Here's how the part is built. I have some questions about the finished solid (model axes, mm). A direction names the side the tool comes from. Give positions to 0.01 mm unless a question says otherwise; leave off trailing zeros. Loops run counter-clockwise (first coordinate to the right, second up) from the corner with the lowest first, then second, coordinate; pieces in that order, holes last. Notation, with made-up numbers: (41.5, 51.5) - (59.5, 51.5) arc R17 ccw to (59.5, 62.5) - close; hole circle Ø2 at (-24.5, -8.5). An arc over 180 degrees is marked (long way). Put each result on its own line as item: value. Start each with the question number.
from build123d import *

# Parameters (mm, degrees)
SKETCH1_R           = 2.5
BOSS_EXTRUDE1_DEPTH = 1
SKETCH2_R           = 1.57
BOSS_EXTRUDE2_DEPTH = 1
BOSS_EXTRUDE3_START = 11
SKETCH3_R           = 2.5
BOSS_EXTRUDE3_DEPTH = 11
SKETCH4_R           = 3
BOSS_EXTRUDE4_DEPTH = 16
SKETCH6_R           = 3.5
BOSS_EXTRUDE6_DEPTH = 8
SKETCH7_W           = 8.052083516
SKETCH7_H           = 1.294876405
CUT_EXTRUDE1_DEPTH  = 30.419381367
SKETCH8_R           = 3.5
BOSS_EXTRUDE7_DEPTH = 29
CUT_EXTRUDE2_START  = -18
SKETCH9_R           = 3
CUT_EXTRUDE2_DEPTH  = 18
SKETCH10_W          = 13
SKETCH10_H          = 5.291502622
CUT_EXTRUDE3_DEPTH  = 3
SKETCH11_R          = 9
BOSS_EXTRUDE8_DEPTH = 4
CUT_EXTRUDE4_START  = -4
SKETCH12_R          = 3
CUT_EXTRUDE4_DEPTH  = 4
CUT_EXTRUDE5_START  = -4
CUT_EXTRUDE5_DEPTH  = 4
SKETCH14_R          = 1
BOSS_EXTRUDE9_DEPTH = 8


with BuildPart() as part:
    # Sketch1 → Boss-Extrude1 (new body)
    with BuildSketch(Plane(origin=(0, 0, 0), x_dir=(0, 0, -1), z_dir=(1, 0, 0))):
        Circle(SKETCH1_R)
    extrude(amount=BOSS_EXTRUDE1_DEPTH)

    # Sketch2 → Boss-Extrude2 (add)
    with BuildSketch(Plane.ZY):
        Circle(SKETCH2_R)
    extrude(amount=BOSS_EXTRUDE2_DEPTH)

    # Sketch3 → Boss-Extrude3 (add)
    with BuildSketch(Plane.ZY.offset(1).offset(BOSS_EXTRUDE3_START)):
        with Locations(Location((0, 0, 0), (0, 0, 180))):
            Circle(SKETCH3_R)
    extrude(amount=-BOSS_EXTRUDE3_DEPTH)

    # Sketch4 → Boss-Extrude4 (add)
    with BuildSketch(Plane.ZY.offset(12)):
        Circle(SKETCH4_R)
    extrude(amount=BOSS_EXTRUDE4_DEPTH)

    # Sketch6 → Boss-Extrude6 (add)
    with BuildSketch(Plane.ZY.offset(28)):
        Circle(SKETCH6_R)
    extrude(amount=BOSS_EXTRUDE6_DEPTH)

    # Sketch7 → Cut-Extrude1 (cut, through all)
    with BuildSketch(Plane(origin=(-28, 0, 0), x_dir=(0, 0, -1), z_dir=(1, 0, 0))):
        with Locations((-0.074496348, 3.647438203)):
            Rectangle(SKETCH7_W, SKETCH7_H)
    extrude(amount=-CUT_EXTRUDE1_DEPTH, mode=Mode.SUBTRACT)

    # Sketch8 → Boss-Extrude7 (add)
    with BuildSketch(Plane.ZY.offset(36)):
        with Locations(Location((0, 0, 0), (0, 0, 121.002719134))):
            Circle(SKETCH8_R)
    extrude(amount=BOSS_EXTRUDE7_DEPTH)

    # Sketch9 → Cut-Extrude2 (cut)
    with BuildSketch(Plane.ZY.offset(65).offset(CUT_EXTRUDE2_START)):
        with Locations(Location((0, 0, 0), (0, 0, 90))):
            Circle(SKETCH9_R)
    extrude(amount=CUT_EXTRUDE2_DEPTH, mode=Mode.SUBTRACT)

    # Sketch10 → Cut-Extrude3 (cut)
    with BuildSketch(Plane(origin=(0, 4, 0), x_dir=(1, 0, 0), z_dir=(0, 1, 0))):
        with Locations((-53.5, 0)):
            Rectangle(SKETCH10_W, SKETCH10_H)
    extrude(amount=-CUT_EXTRUDE3_DEPTH, mode=Mode.SUBTRACT)

    # Sketch11 → Boss-Extrude8 (add)
    with BuildSketch(Plane.ZY.offset(65)):
        Circle(SKETCH11_R)
    extrude(amount=BOSS_EXTRUDE8_DEPTH)

    # Sketch12 → Cut-Extrude4 (cut)
    with BuildSketch(Plane.ZY.offset(69).offset(CUT_EXTRUDE4_START)):
        with Locations(Location((0, 0, 0), (0, 0, 90))):
            Circle(SKETCH12_R)
    extrude(amount=CUT_EXTRUDE4_DEPTH, mode=Mode.SUBTRACT)

    # Sketch13 → Cut-Extrude5 (cut)
    with BuildSketch(Plane.ZY.offset(69).offset(CUT_EXTRUDE5_START)):
        with BuildLine():
            ThreePointArc((-2.5, 8.645808233), (-7.193747285, 5.408326913), (-9, 0))
            Line((-9, 0), (-5, 0))
            Line((-5, 0), (-2.5, 8.645808233))
        make_face()
        with BuildLine():
            Line((5, 0), (9, 0))
            ThreePointArc((9, 0), (7.193747285, 5.408326913), (2.5, 8.645808233))
            Line((2.5, 8.645808233), (5, 0))
        make_face()
    extrude(amount=CUT_EXTRUDE5_DEPTH, mode=Mode.SUBTRACT)

    # Sketch14 → Boss-Extrude9 (add)
    with BuildSketch(Plane.ZY.offset(69)):
        with Locations(Location((0, 8, 0), (0, 0, 89.999140318))):
            Circle(SKETCH14_R)
    extrude(amount=BOSS_EXTRUDE9_DEPTH)


solid = part.part
1) Suppose I cut it at A-A on x = -56.5. Please give me the cut outline in (y, z).
2) Suppose I cut it at B-B on y = -6.5. Please give me the cut outline in (x, z), plus the area to 3 significant figures.
3) I'm going to push flat-ended pins straight in: P1, Ø1, axis at x = -53, y = 2, coming from the +Z side; P2, Ø1.1, axis at x = -32.5, z = 0, coming from the +Y side; P3, Ø3, axis at y = -3, z = 3, coming from the +X side. Where does each tip first touch, or does it pass through?
4) Which directions (+Z, -Z, +X, -X, +Y, -Y) give clear straight access to the entire face, cutting with the end or side of a thin tool? Please do faces 1 (the flat face through (-67, 0, 7)), 2 (the flat face through (0, -2, 0)), 3 (the flat face through (-65, -4, 0)).
5) I need wall thicknesses on line 1 (Z direction, x = -63.25, y = 0); line 2 (X direction, y = 3.25, z = -1); line 3 (X direction, y = 7.5, z = -1.25). Which ranges of each line are inside material? Lowest first, please.
6) Thinking about a two-plate mould opening in X: for faces 4 (the flat face through (-1, 2, 0)), 5 (the flat face through (-12, 2, -2)), 6 (the cylindrical face through (-73, 7, 0)), which applies, pulls with the +X half, pulls with the -X half, needs draft (parallel to the pull), parting line crosses it, or undercut?
Ans:
1. outline: (1.41, -2.65) arc R3 cw (long way) to (1.41, 2.65) - (2.29, 2.65) arc R3.5 ccw (long way) to (2.29, -2.65) - close
2. outline: (-69, -6.22) - (-65, -6.22) - (-65, 6.22) - (-69, 6.22) - close
2. area: 49.8 mm²
3. P1: stops at z = 3.16
3. P2: stops at y = 3
3. P3: stops at x = -12
4. face 1: +Z, +X, -X, +Y
4. face 2: none
4. face 3: +X
5. line 1: z = -3.5 to -3, 3 to 3.5
5. line 2: x = -69 to -60, -47 to -36
5. line 3: x = -69 to -65
6. face 4: undercut
6. face 5: pulls with the +X half
6. face 6: needs draft
